```python
from build123d import *

# Parameters (mm, degrees)
PAD_DEPTH       = 20
SKETCH001_R     = 1.7
POCKET_DEPTH    = 5
SKETCH002_R     = 1.7
POCKET001_DEPTH = 5
SKETCH003_R     = 1.7
SKETCH003_W     = 21
SKETCH003_H     = 2.5
POCKET002_DEPTH = 9
SKETCH004_R     = 3.2
POCKET003_DEPTH = 3
SKETCH005_R     = 3.2
POCKET004_DEPTH = 3
SKETCH006_R     = 3.2
POCKET005_DEPTH = 3


with BuildPart() as part:
    # Sketch → Pad (new body)
    with BuildSketch(Plane.XY):
        Polygon((-2, 22), (2, 22), (2, 2), (22, 2), (22, -2), (3.065041, -2), (-23.92031, -28.985351), (-35.234019, -28.985351), (-2, 4.248668), align=None)
    extrude(amount=PAD_DEPTH)

    # Sketch001 (on Face2 of Pad) → Pocket (cut)
    with BuildSketch(Plane(origin=(-2, 0, 0), x_dir=(0, -1, 0), z_dir=(-1, 0, 0))):
        with Locations((-12, 10)):
            Circle(SKETCH001_R)
    extrude(amount=-POCKET_DEPTH, mode=Mode.SUBTRACT)

    # Sketch002 (on Face12 of Pocket) → Pocket001 (cut)
    with BuildSketch(Plane.XZ.offset(2)):
        with Locations((12, 10)):
            Circle(SKETCH002_R)
    extrude(amount=-POCKET001_DEPTH, mode=Mode.SUBTRACT)

    # Sketch003 (on Face1 of Pocket001) → Pocket002 (cut)
    with BuildSketch(Plane(origin=(-3.124334, 3.124334, 0), x_dir=(-0.707107, -0.707107, 0), z_dir=(-0.707107, 0.707107, 0))):
        with Locations((17.409952, 10)):
            Circle(SKETCH003_R)
        with Locations((26.409952, 10)):
            Circle(SKETCH003_R)
        with Locations((22.409952, 1.25)):
            Rectangle(SKETCH003_W, SKETCH003_H)
    extrude(amount=-POCKET002_DEPTH, mode=Mode.SUBTRACT)

    # Sketch004 (on Face7 of Pocket002) → Pocket003 (cut)
    with BuildSketch(Plane(origin=(-2, 0, 0), x_dir=(0, -1, 0), z_dir=(-1, 0, 0))):
        with Locations((-12, 10)):
            Circle(SKETCH004_R)
    extrude(amount=-POCKET003_DEPTH, mode=Mode.SUBTRACT)

    # Sketch005 (on Face13 of Pocket003) → Pocket004 (cut)
    with BuildSketch(Plane.XZ.offset(2)):
        with Locations((12, 10)):
            Circle(SKETCH005_R)
    extrude(amount=-POCKET004_DEPTH, mode=Mode.SUBTRACT)

    # Sketch006 (on Face1 of Pocket004) → Pocket005 (cut)
    with BuildSketch(Plane(origin=(-3.124334, 3.124334, 0), x_dir=(-0.707107, -0.707107, 0), z_dir=(-0.707107, 0.707107, 0))):
        with Locations((17.409955, 10.000001)):
            Circle(SKETCH006_R)
        with Locations((26.368249, 9.834363)):
            Circle(SKETCH006_R)
    extrude(amount=-POCKET005_DEPTH, mode=Mode.SUBTRACT)


solid = part.part
```
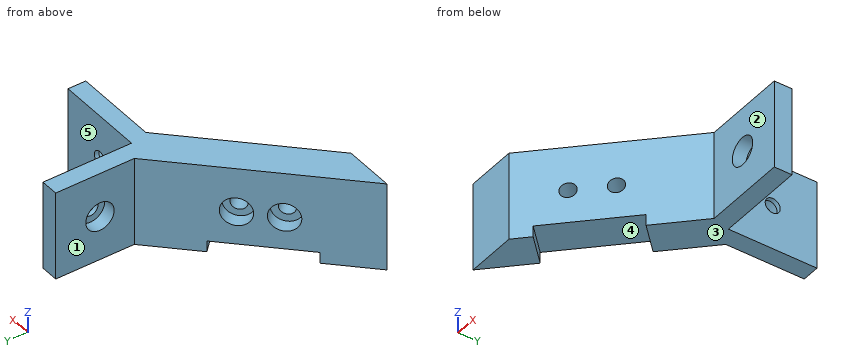
Work out the finished part from the listing and answer in its coordinate system (mm). Face numbers are marked on the shaded views. A direction names the side the tool comes from. Round coordinates to 2 decimals unless told otherwise and drop trailing zeros. Write each loop counter-clockwise with the first axis right and the second up, starting at its lowest first coordinate (ties: lowest second). Pieces come first, ordered by that corner, then holes. Notation, with made-up numbers: (-13, 66) - (38, 66) arc R30 ccw to (38, 97) - close; hole circle Ø10 at (70, 9). An arc over 180 degrees is marked (long way). Return JSON: item names as keys, results as strings. Group by question number.
Q1. The part is cut by section C-C on z = 17. Write down the section's boundary in (x, y).
Q2. For the marked faces 1, 2, 3, 4 and 5, determine the directions among +Z, -Z, +X, -X, +Y, -Y from which every point of the face is accessible in a straight line to the end or side of a thin tool.
Q3. The part is cut by section D-D on x = -7.5. Write down the section's boundary in (y, z).
Q4. The part is cut by section A-A on y = 12. Write down the section's boundary in (x, z).
Q5. Each of these flat-tipped pins is pushed along its axis until it touches: pin 1 Ø5 at (y, z) = (11.5, 9) entering from -X; pin 2 Ø8 at (y, z) = (-18.5, 9) entering from -X; pin 3 Ø4 at (y, z) = (12, 10) entering from +X. Where does it stop, or does it pass through?
Q6. Find the intervals of material crossed by L1, parallel to Z at x = -0.75, y = 12; L2, parallel to Z at x = 1.3, y = 12; L3, parallel to X at y = 17, z = 10.25, in increasing order.
Solved:
{
 "1": {"outline": "(-35.23, -28.99) - (-23.92, -28.99) - (3.07, -2) - (22, -2) - (22, 2) - (2, 2) - (2, 22) - (-2, 22) - (-2, 4.25) - close"},
 "2": {"face 1": "+Z, -Z, -X, +Y", "face 2": "+Z, -Z, +X, -Y", "face 3": "-Z, +X, -X, +Y, -Y", "face 4": "-Z", "face 5": "+Z, -Z, +X, +Y"},
 "3": {"outline": "(-12.57, 2.5) - (-9.34, 2.5) - (-9.34, 0) - (-1.25, 0) - (-1.25, 20) - (-12.57, 20) - close"},
 "4": {"outline": "(-2, 0) - (2, 0) - (2, 8.3) - (1, 8.3) - (1, 6.8) - (-2, 6.8) - close; (-2, 13.2) - (1, 13.2) - (1, 11.7) - (2, 11.7) - (2, 20) - (-2, 20) - close"},
 "5": {"pin 1": "x = -2", "pin 2": "x = -28.75", "pin 3": "x = 2"},
 "6": {"L1": "0 to 6.8, 13.2 to 20", "L2": "0 to 8.3, 11.7 to 20", "L3": "-2 to 2"}
}
